Geometry: final body of the model. Coordinates: model frame, mm. Face numbers are marked on the shaded views. A direction names the side the tool comes from. Give positions to 0.01 mm unless a question says otherwise; leave off trailing zeros. Write each loop counter-clockwise with the first axis right and the second up, starting at its lowest first coordinate (ties: lowest second). Pieces come first, ordered by that corner, then holes. Notation, with made-up numbers: (39.5, 63) - (85.5, 63) arc R18 ccw to (85.5, 81) - close; hole circle Ø3 at (8, 20). An arc over 180 degrees is marked (long way). Use CSV: the item, a comma, the result in double quotes. Start each with the question number.
(1) Line query: probe 1 along Y at (x, z) = (7.75, 0.55); probe 2 along X at (y, z) = (2.5, 3.75); probe 3 along X at (y, z) = (2.75, -0.25). Output: solid intervals per line, ascending. Write a range as [from, to].
(2) Draft query along Y for the marked faces 6, 7, 8 and 9. Return one class per face: released by +Y, released by -Y, zero draft, split by the parting line, or undercut.
(3) Section A-A on x = 7.75. Output: boundary loops of the cut face in (y, z).
(4) Reachability of the marked faces 1, 2, 3, 4 and 5 from +Z, -Z, +X, -X, +Y, -Y: full face, straight path, thin tool, end or side. Return the list, or none.
(5) First-contact query: pin 1 Ø1.4 at (y, z) = (2, 5.5) entering from +X; pin 2 Ø2.5 at (y, z) = (3, 3.5) entering from -X; pin 3 Ø2 at (x, y) = (1.5, 4.5) entering from -Z. Flat tips, straight axial feed; report the tip coordinate or a pass-through.
(6) Section C-C on y = 9.75. Output: boundary loops of the cut face in (x, z), and give its area (4 significant figures).
(7) Section D-D on y = 15. Output: boundary loops of the cut face in (x, z), and give its area (3 significant figures).
(8) Section B-B on z = 4.5. Output: boundary loops of the cut face in (x, y).
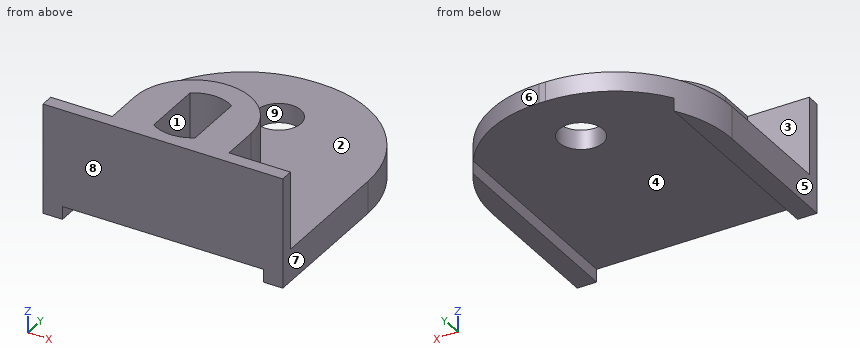
from build123d import *

# Parameters (mm, degrees)
EXTRUDE_1_DEPTH     = 20
FILLET_1_R          = 9
SKETCH_2_R          = 1.7
CUT_EXTRUDE_1_DEPTH = 3.5
SKETCH_3_W          = 18.5
SKETCH_3_H          = 1
EXTRUDE_2_DEPTH     = 6
EXTRUDE_3_DEPTH     = 6


with BuildPart() as part:
    # Эскиз1 → Бобышка-Вытянуть1 (new body)
    with BuildSketch(Plane(origin=(0, 0, 0), x_dir=(1, 0, 0), z_dir=(0, 1, 0))):
        Polygon((0, 0), (15.5, 0), (15.5, 1), (17, 1), (17, -1.5), (-1.5, -1.5), (-1.5, 1), (0, 1), align=None)
    extrude(amount=EXTRUDE_1_DEPTH)

    # Скругление1
    fillet_1_edges = [part.edges().sort_by_distance(p)[0] for p in [
        (-1.5, 20, 0.25),
        (17, 20, 0.25),
    ]]
    fillet(fillet_1_edges, radius=FILLET_1_R)

    # Эскиз2 → Вырез-Вытянуть1 (cut, through all)
    with BuildSketch(Plane.XY.offset(1.5)):
        with Locations((7.75, 15)):
            Circle(SKETCH_2_R)
    extrude(amount=-CUT_EXTRUDE_1_DEPTH, mode=Mode.SUBTRACT)

    # Эскиз3 → Бобышка-Вытянуть2 (add)
    with BuildSketch(Plane.XY.offset(1.5)):
        with Locations((7.75, 0.5)):
            Rectangle(SKETCH_3_W, SKETCH_3_H)
    extrude(amount=EXTRUDE_2_DEPTH)

    # Эскиз4 → Бобышка-Вытянуть3 (add)
    with BuildSketch(Plane.XY.offset(1.5)):
        with BuildLine():
            Line((3.25, 3.85), (3.25, 1.023796375))
            Line((3.25, 1.023796375), (3.25, 0.775352043))
            Line((3.25, 0.775352043), (12.25, 0.775352043))
            Line((12.25, 0.775352043), (12.25, 1.023796375))
            Line((12.25, 1.023796375), (12.25, 3.85))
            ThreePointArc((12.25, 3.85), (7.75, 8.35), (3.25, 3.85))
        make_face()
        with BuildLine():
            Line((6.15, 6.208495283), (6.15, 1.491504717))
            ThreePointArc((6.15, 1.491504717), (7.75, 1), (9.35, 1.491504717))
            Line((9.35, 1.491504717), (9.35, 6.208495283))
            ThreePointArc((9.35, 6.208495283), (7.75, 6.7), (6.15, 6.208495283))
        make_face(mode=Mode.SUBTRACT)
    extrude(amount=EXTRUDE_3_DEPTH)


solid = part.part
Check values:
1,probe 1,"y = [0, 13.3], [16.7, 20]"
1,probe 2,"x = [3.25, 6.15], [9.35, 12.25]"
1,probe 3,"x = [-1.5, 0], [15.5, 17]"
2,face 6,"released by +Y"
2,face 7,"zero draft"
2,face 8,"released by -Y"
2,face 9,"undercut"
3,outline,"(0, 0) - (13.3, 0) - (13.3, 1.5) - (8.35, 1.5) - (8.35, 7.5) - (6.7, 7.5) - (6.7, 1.5) - (1, 1.5) - (1, 7.5) - (0, 7.5) - close; (16.7, 0) - (20, 0) - (20, 1.5) - (16.7, 1.5) - close"
4,face 1,"+Z"
4,face 2,"+Z, +Y"
4,face 3,"+Z, -X, +Y"
4,face 4,"-Z, +Y, -Y"
4,face 5,"+Z, -Z, -X, +Y, -Y"
5,pin 1,"stops at x = 12.25"
5,pin 2,"stops at x = 3.25"
5,pin 3,"stops at z = 0"
6,outline,"(-1.5, -1) - (0, -1) - (0, 0) - (15.5, 0) - (15.5, -1) - (17, -1) - (17, 1.5) - (-1.5, 1.5) - close"
6,area,"30.75 mm²"
7,outline,"(-0.56, -1) - (0, -1) - (0, 0) - (6.05, 0) - (6.05, 1.5) - (-0.56, 1.5) - close; (9.45, 0) - (15.5, 0) - (15.5, -1) - (16.06, -1) - (16.06, 1.5) - (9.45, 1.5) - close"
7,area,"21.0 mm²"
8,outline,"(-1.5, 0) - (17, 0) - (17, 1) - (12.25, 1) - (12.25, 3.85) arc R4.5 ccw to (3.25, 3.85) - (3.25, 1) - (-1.5, 1) - close; hole (6.15, 1.49) arc R2.85 ccw to (9.35, 1.49) - (9.35, 6.21) arc R2.85 ccw to (6.15, 6.21) - close"
